CAD build for the part. Positions are in the model's coordinates, mm. A direction names the side the tool comes from. Give positions to 0.01 mm unless a question says otherwise; leave off trailing zeros. Write each loop counter-clockwise with the first axis right and the second up, starting at its lowest first coordinate (ties: lowest second). Pieces come first, ordered by that corner, then holes. Notation, with made-up numbers: (86.5, 88) - (99.5, 88) arc R9 cw to (99.5, 93) - close; hole circle Ø8 at (51, 25.5). An arc over 180 degrees is marked (long way). Write item = value, one per line. Start each with the question number.
```python
from build123d import *

# Parameters (mm, degrees)
SKETCH3_R                 = 2.75
BOSS_EXTRUDE1_DEPTH       = 6
BOSS_EXTRUDE1_2_DEPTH     = 6
BOSS_EXTRUDE1_3_DEPTH     = 6
BOSS_EXTRUDE1_4_DEPTH     = 6
SKETCH4_W                 = 43
SKETCH4_H                 = 86
BOSS_EXTRUDE2_DEPTH       = 2.5
SKETCH5_R                 = 2.75
BOSS_EXTRUDE3_DEPTH       = 10
LPATTERN1_COUNT           = 2
LPATTERN1_PITCH           = 37
LPATTERN2_COUNT           = 2
LPATTERN2_PITCH           = 37
LPATTERN2_COPY_1_SKETCH_R = 2.75
LPATTERN2_COPY_1_DEPTH    = 10
SKETCH6_W                 = 87
SKETCH6_H                 = 86
BOSS_EXTRUDE4_DEPTH       = 2.5
BOSS_EXTRUDE5_DEPTH       = 2
SKETCH12_W                = 4
SKETCH12_H                = 8
CUT_EXTRUDE1_DEPTH        = 4
SKETCH14_R                = 0.85
CUT_EXTRUDE2_DEPTH        = 4.5
LPATTERN3_COUNT           = 2
LPATTERN3_PITCH           = 46.5
BOSS_EXTRUDE6_DEPTH       = 35
SKETCH18_W                = 2
SKETCH18_H                = 35
BOSS_EXTRUDE7_DEPTH       = 18.5
SKETCH19_W                = 32.48
SKETCH19_H                = 17.04
BOSS_EXTRUDE8_DEPTH       = 10
SKETCH20_W                = 8.16
SKETCH20_H                = 13.04
CUT_EXTRUDE3_DEPTH        = 10
SKETCH21_W                = 1.1
SKETCH21_H                = 86
CUT_EXTRUDE4_DEPTH        = 10
FILLET2_R                 = 2
FILLET4_R                 = 20
BOSS_EXTRUDE9_DEPTH       = 2.5
SKETCH24_W                = 10
SKETCH24_H                = 20
BOSS_EXTRUDE10_DEPTH      = 30
SKETCH25_R                = 5
CUT_EXTRUDE6_DEPTH        = 30
FILLET6_R                 = 10
FILLET8_R                 = 2
SKETCH27_W                = 20
SKETCH27_H                = 20.130693805
CUT_EXTRUDE7_DEPTH        = 22.5
CUT_EXTRUDE10_DEPTH       = 7.5
CUT_EXTRUDE10_DEPTH_BACK  = 210.5
SKETCH28_W                = 79.126815109
SKETCH28_H                = 112.332596714
SKETCH29_R                = 1.25
CUT_EXTRUDE11_DEPTH       = 19.5
SKETCH30_W                = 10
SKETCH30_H                = 5
CUT_EXTRUDE12_DEPTH       = 4.5
FILLET9_R                 = 5
FILLET9_OF_MIRROR5_R      = 5
FILLET11_R                = 1


with BuildPart() as part:
    # Sketch3 → Boss-Extrude1 (new body)
    with BuildSketch(Plane.XY):
        with Locations((-25, -3)):
            Circle(SKETCH3_R)
    boss_extrude1 = extrude(amount=BOSS_EXTRUDE1_DEPTH)



with BuildPart() as body_2:
    # Sketch3 → Boss-Extrude1 2 (new body)
    with BuildSketch(Plane.XY):
        with Locations((-62, -3)):
            Circle(SKETCH3_R)
    boss_extrude1_2 = extrude(amount=BOSS_EXTRUDE1_2_DEPTH)


with BuildPart() as body_3:
    # Sketch3 → Boss-Extrude1 3 (new body)
    with BuildSketch(Plane.XY):
        with Locations(Location((-25, -40, 0), (0, 0, 180))):
            Circle(SKETCH3_R)
    boss_extrude1_3 = extrude(amount=BOSS_EXTRUDE1_3_DEPTH)


with BuildPart() as body_4:
    # Sketch3 → Boss-Extrude1 4 (new body)
    with BuildSketch(Plane.XY):
        with Locations(Location((-62, -40, 0), (0, 0, 180))):
            Circle(SKETCH3_R)
    boss_extrude1_4 = extrude(amount=BOSS_EXTRUDE1_4_DEPTH)


with BuildPart() as part_1:
    add(part.part)

    add(body_2.part)  # Boss-Extrude2 merges body 2

    add(body_3.part)  # Boss-Extrude2 merges body 3

    add(body_4.part)  # Boss-Extrude2 merges body 4
    # Sketch4 → Boss-Extrude2 (add)
    with BuildSketch(Plane.XY):
        with Locations((-43.5, 0)):
            Rectangle(SKETCH4_W, SKETCH4_H)
    extrude(amount=-BOSS_EXTRUDE2_DEPTH)

    # Mirror4: Boss-Extrude1, Boss-Extrude1 2, Boss-Extrude1 3, Boss-Extrude1 4 across plane
    add(boss_extrude1.mirror(Plane.ZX))
    add(boss_extrude1_2.mirror(Plane.ZX))
    add(boss_extrude1_3.mirror(Plane.ZX))
    add(boss_extrude1_4.mirror(Plane.ZX))

    # Sketch5 → Boss-Extrude3 (add)
    with BuildSketch(Plane.XY.offset(6)):
        with Locations((-25, 40)):
            Circle(SKETCH5_R)
    boss_extrude3 = extrude(amount=BOSS_EXTRUDE3_DEPTH)

    # LPattern1: Boss-Extrude3 ×2
    with Locations(*[(-i * LPATTERN1_PITCH, 0, 0) for i in range(1, LPATTERN1_COUNT)]):
        add(boss_extrude3)

    # LPattern2: Boss-Extrude3 ×2
    with Locations(*[(0, -i * LPATTERN2_PITCH, 0) for i in range(1, LPATTERN2_COUNT)]):
        add(boss_extrude3)

    # LPattern2 copy 1 sketch → LPattern2 copy 1 (add)
    with BuildSketch(Plane(origin=(-37, -37, 6), x_dir=(1, 0, 0), z_dir=(0, 0, 1))):
        with Locations((-25, 40)):
            Circle(LPATTERN2_COPY_1_SKETCH_R)
    extrude(amount=LPATTERN2_COPY_1_DEPTH)

    # Sketch6 → Boss-Extrude4 (add)
    with BuildSketch(Plane.XY):
        with Locations((21.5, 0)):
            Rectangle(SKETCH6_W, SKETCH6_H)
    extrude(amount=-BOSS_EXTRUDE4_DEPTH)

    # Sketch11 → Boss-Extrude5 (add, symmetric)
    with BuildSketch(Plane(origin=(-6, 0, 0), x_dir=(0, 0, -1), z_dir=(1, 0, 0))):
        Polygon((0, -43), (-40, -43), (-40, -39), (0, -18), align=None)
    boss_extrude5 = extrude(amount=BOSS_EXTRUDE5_DEPTH, both=True)

    # Sketch12 → Cut-Extrude1 (cut)
    with BuildSketch(Plane.ZY.offset(8)):
        with Locations((8, -32)):
            Rectangle(SKETCH12_W, SKETCH12_H)
    extrude(amount=-CUT_EXTRUDE1_DEPTH, mode=Mode.SUBTRACT)

    # Sketch14 → Cut-Extrude2 (cut)
    with BuildSketch(Plane.XZ.offset(43)):
        with Locations(Location((-6, 37, 0), (0, 0, 270))):
            Circle(SKETCH14_R)
        with Locations(Location((-6, 13.6, 0), (0, 0, 270))):
            Circle(SKETCH14_R)
    cut_extrude2 = extrude(amount=-CUT_EXTRUDE2_DEPTH, mode=Mode.SUBTRACT)

    # LPattern3: Boss-Extrude5, Cut-Extrude2 ×2
    with Locations(*[(i * LPATTERN3_PITCH, 0, 0) for i in range(1, LPATTERN3_COUNT)]):
        add(boss_extrude5)
        add(cut_extrude2, mode=Mode.SUBTRACT)

    # Sketch17 → Boss-Extrude6 (add)
    with BuildSketch(Plane.XY):
        Polygon((42.5, -41), (42.5, -43), (63.9, -43), (63.9, 25.4), (40.5, 25.4), (40.5, -18), (42.5, -18), (42.5, 23.4), (61.9, 23.4), (61.9, -41), align=None)
    extrude(amount=BOSS_EXTRUDE6_DEPTH)

    # Sketch18 → Boss-Extrude7 (add)
    with BuildSketch(Plane.XZ.offset(18)):
        with Locations((41.5, 17.5)):
            Rectangle(SKETCH18_W, SKETCH18_H)
    extrude(amount=BOSS_EXTRUDE7_DEPTH)

    # Sketch19 → Boss-Extrude8 (add)
    with BuildSketch(Plane.XY):
        with Locations((16.24, 8.52)):
            Rectangle(SKETCH19_W, SKETCH19_H)
    extrude(amount=BOSS_EXTRUDE8_DEPTH)

    # Sketch20 → Cut-Extrude3 (cut)
    with BuildSketch(Plane.XY.offset(10)):
        with Locations((6.08, 8.52)):
            Rectangle(SKETCH20_W, SKETCH20_H)
        with Locations((16.24, 8.52)):
            Rectangle(SKETCH20_W, SKETCH20_H)
        with Locations((26.4, 8.52)):
            Rectangle(SKETCH20_W, SKETCH20_H)
    extrude(amount=-CUT_EXTRUDE3_DEPTH, mode=Mode.SUBTRACT)

    # Sketch21 → Cut-Extrude4 (cut)
    with BuildSketch(Plane.XY):
        with Locations((64.45, 0)):
            Rectangle(SKETCH21_W, SKETCH21_H)
    extrude(amount=-CUT_EXTRUDE4_DEPTH, mode=Mode.SUBTRACT)

    # Fillet2
    fillet2_edges = [part_1.edges().sort_by_distance(p)[0] for p in [
        (63.9, -43, 16.25),
        (63.9, 25.4, 17.5),
        (-65, -43, -1.25),
        (-65, 43, -1.25),
    ]]
    fillet(fillet2_edges, radius=FILLET2_R)

    # Fillet4
    fillet4_edges = [part_1.edges().sort_by_distance(p)[0] for p in [
        (63.9, 43, -1.25),
    ]]
    fillet(fillet4_edges, radius=FILLET4_R)

    # Sketch23 → Boss-Extrude9 (add)
    with BuildSketch(Plane(origin=(0, 0, -2.5), x_dir=(-1, 0, 0), z_dir=(0, 0, -1))):
        with BuildLine():
            Line((95.480174176, -10), (105, -10))
            Line((105, -10), (110, -10))
            Line((110, -10), (110, 10))
            Line((110, 10), (105, 10))
            Line((105, 10), (95.480174176, 10))
            add(Edge.make_bspline(
                [(95.480174176, 10), (68.262963787, 8.86232235), (65, 41)],
                knots=[0, 0, 0, 1, 1, 1], degree=2))
            Line((65, 41), (65, -41))
            add(Edge.make_bspline(
                [(95.480174176, -10), (68.262963787, -8.86232235), (65, -41)],
                knots=[0, 0, 0, 1, 1, 1], degree=2))
        make_face()
    extrude(amount=-BOSS_EXTRUDE9_DEPTH)

    # Sketch24 → Boss-Extrude10 (add)
    with BuildSketch(Plane.XY):
        with Locations((-105, 0)):
            Rectangle(SKETCH24_W, SKETCH24_H)
    extrude(amount=BOSS_EXTRUDE10_DEPTH)

    # Sketch25 → Cut-Extrude6 (cut)
    with BuildSketch(Plane.ZY.offset(110)):
        with Locations((20, 0)):
            Circle(SKETCH25_R)
    extrude(amount=-CUT_EXTRUDE6_DEPTH, mode=Mode.SUBTRACT)

    # Fillet6
    fillet6_edges = [part_1.edges().sort_by_distance(p)[0] for p in [
        (-100, 0, 0),
    ]]
    fillet(fillet6_edges, radius=FILLET6_R)

    # Fillet8
    fillet8_edges = [part_1.edges().sort_by_distance(p)[0] for p in [
        (-110, 10, 15),
        (-110, -10, 15),
    ]]
    fillet(fillet8_edges, radius=FILLET8_R)

    # Sketch27 → Cut-Extrude7 (cut)
    with BuildSketch(Plane(origin=(0, 0, -2.5), x_dir=(-1, 0, 0), z_dir=(0, 0, -1))):
        with Locations((100, -0.065346902)):
            Rectangle(SKETCH27_W, SKETCH27_H)
    extrude(amount=-CUT_EXTRUDE7_DEPTH, mode=Mode.SUBTRACT)


with BuildPart() as cut_extrude7_piece_1:
    # of the separate pieces the step leaves, piece 1, a body of its own (cut_extrude7_pieces)
    add(part_1.part.solids().sort_by_distance((-90, -10.130693805, -2.5))[0])

    # Sketch28 → Cut-Extrude10 (cut, two sides: drawn at the far end of the back side and taken through both)
    with BuildSketch(Plane.ZY.offset(90).offset(-CUT_EXTRUDE10_DEPTH_BACK)):
        with Locations((27.34304702, -0.64713832)):
            Rectangle(SKETCH28_W, SKETCH28_H)
    extrude(amount=CUT_EXTRUDE10_DEPTH + CUT_EXTRUDE10_DEPTH_BACK, mode=Mode.SUBTRACT)


with BuildPart() as cut_extrude7_piece_2:
    # of the separate pieces the step leaves, piece 2, a body of its own (cut_extrude7_pieces)
    add(part_1.part.solids().sort_by_distance((-108, 10, 20))[0])

    # Sketch29 → Cut-Extrude11 (cut)
    with BuildSketch(Plane(origin=(0, 0, 20), x_dir=(-1, 0, 0), z_dir=(0, 0, -1))):
        with Locations((105, 7.5)):
            Circle(SKETCH29_R)
    cut_extrude11 = extrude(amount=-CUT_EXTRUDE11_DEPTH, mode=Mode.SUBTRACT)

    # Sketch30 → Cut-Extrude12 (cut)
    with BuildSketch(Plane.XY.offset(30)):
        with Locations((-105, 7.5)):
            Rectangle(SKETCH30_W, SKETCH30_H)
    cut_extrude12 = extrude(amount=-CUT_EXTRUDE12_DEPTH, mode=Mode.SUBTRACT)

    # Fillet9
    # the kernel refuses this fillet: 5 mm, written as the material it takes off along each edge
    with BuildSketch(Plane(origin=(-122.437342964, 5, 30), x_dir=(0, -1, 0), z_dir=(1, 0, 0))) as fillet9_piece_1:
        with BuildLine():
            CenterArc((4.974937186, 5), FILLET9_R, 185.739170477, 84.260829523)
            Line((0, 4.5), (-0.099498744, 4.49))
            ThreePointArc((-0.099498744, 4.49), (-0.1, 2.25), (-0.1, 0))
            Line((-0.1, 0), (0, -0.1))
            Line((0, -0.1), (4.974937186, -0.1))
            Line((4.974937186, -0.1), (4.974937186, 0))
        make_face()
    extrude(amount=34.874685928, mode=Mode.SUBTRACT)

    # Mirror5: Cut-Extrude11, Cut-Extrude12 across plane
    add(cut_extrude11.mirror(Plane.ZX), mode=Mode.SUBTRACT)
    add(cut_extrude12.mirror(Plane.ZX), mode=Mode.SUBTRACT)

    # Fillet9 of Mirror5
    # the kernel refuses this fillet: 5 mm, written as the material it takes off along each edge
    with BuildSketch(Plane(origin=(-122.437342964, -5, 30), x_dir=(0, 0, -1), z_dir=(1, 0, 0))) as fillet9_of_mirror5_piece_1:
        with BuildLine():
            CenterArc((5, 4.974937186), FILLET9_OF_MIRROR5_R, 180, 84.260829523)
            Line((0, 4.974937186), (-0.1, 4.974937186))
            Line((-0.1, 4.974937186), (-0.1, 0))
            Line((-0.1, 0), (0, -0.1))
            ThreePointArc((0, -0.1), (2.25, -0.1), (4.49, -0.099498744))
            Line((4.49, -0.099498744), (4.5, 0))
        make_face()
    extrude(amount=34.874685928, mode=Mode.SUBTRACT)

    # Fillet11
    fillet11_edges = [cut_extrude7_piece_2.edges().sort_by_distance(p)[0] for p in [
        (-104, 10, 25.5),
        (-109.414213562, 9.414213562, 25.5),
        (-110, 6.5, 25.5),
        (-100, 7.5, 25.5),
        (-100, 3.379164781, 28.708099244),
        (-110, 0, 30),
        (-110, 3.379164781, 28.708099244),
        (-109.414213562, -9.414213562, 25.5),
        (-110, -6.5, 25.5),
        (-100, -7.5, 25.5),
        (-104, -10, 25.5),
        (-100, 0, 30),
        (-100, -3.379164781, 28.708099244),
        (-110, -3.379164781, 28.708099244),
    ]]
    fillet(fillet11_edges, radius=FILLET11_R)


solid = cut_extrude7_piece_2.part
```
1. Tool access for faces 4 (the flat face through (-105, 6, 25.5)), 5 (the cylindrical face through (-100.285, -7.039, 25.199)), 6 (the cylindrical face through (-109.699, -6.47, 25.215)): list every direction of +Z, -Z, +X, -X, +Y, -Y with a clear straight run to the whole face (end or side of a thin tool).
2. Cut at A-A (x = -105). Give the cut face in (y, z), then the cut area to 3 significant figures.
3. Cut at D-D (y = -5.75). Give the cut face in (x, z).
4. Mould opens along Y. For faces 1 (the flat face through (-104, 6, 20)), 2 (the cylindrical face through (-105.06, 3.42, 28.67)), 3 (the cylindrical face through (-106.155, 7.021, 22.712)) say: +Y half, -Y half, draft (parallel to the pull), parting line (faces both ways), or undercut.
5. Pin check, flat tips, straight feed: pin 1 Ø1.5 at (x, z) = (-108.5, 28) entering from +Y; pin 2 Ø3 at (x, y) = (-105, 7.5) entering from +Z; pin 3 Ø1.5 at (y, z) = (-7, 27.5) entering from +X. Stop position of each tip, or through.
6. Cut at C-C (x = -103.25). Give the cut face in (y, z), then the cut area to 3 significant figures.
7. Cut at B-B (y = 7.5). Give the cut face in (x, z).
8. Wall check: line 1 along Y through (x, z) = (-105, 23.05); line 2 along Y through (x, z) = (-105, 24); line 3 along Z through (x, y) = (-104.25, -6). Give the ranges that are in metal, low to high.
Output:
q1.face_4 = +Z, +X, -X, +Y
q1.face_5 = +Z, +X, -Y
q1.face_6 = +Z, -X, -Y
q2.outline = (-10, 20) - (-8.75, 20) - (-8.75, 25.5) - (-9, 25.5) arc R1 ccw to (-10, 24.5) - close; (-6.25, 20) - (-5, 20) arc R5 cw to (5, 20) - (6.25, 20) - (6.25, 25.5) - (5, 25.5) arc R5 ccw to (0.03, 30) - (-0.03, 30) arc R5 ccw to (-5, 25.5) - (-6.25, 25.5) - close; (8.75, 20) - (10, 20) - (10, 24.5) arc R1 ccw to (9, 25.5) - (8.75, 25.5) - close
q2.area = 77.3 mm2
q3.outline = (-110, 20) - (-100, 20) - (-100, 24.5) arc R1 ccw to (-101, 25.5) - (-109, 25.5) arc R1 ccw to (-110, 24.5) - close
q4.face_1 = draft
q4.face_2 = +Y half
q4.face_3 = undercut
q5.pin_1 = 4.49
q5.pin_2 = 25.5
q5.pin_3 = through
q6.outline = (-10, 20) - (-5, 20) arc R5 cw to (5, 20) - (10, 20) - (10, 24.5) arc R1 ccw to (9, 25.5) - (5, 25.5) arc R5 ccw to (0.03, 30) - (-0.03, 30) arc R5 ccw to (-5, 25.5) - (-9, 25.5) arc R1 ccw to (-10, 24.5) - close
q6.area = 105 mm2
q7.outline = (-110, 20) - (-106.25, 20) - (-106.25, 25.5) - (-109, 25.5) arc R1 ccw to (-110, 24.5) - close; (-103.75, 20) - (-100, 20) - (-100, 24.5) arc R1 ccw to (-101, 25.5) - (-103.75, 25.5) - close
q8.line_1 = -10 to -8.75, -6.25 to -3.96, 3.96 to 6.25, 8.75 to 10
q8.line_2 = -10 to -8.75, -6.25 to -3, 3 to 6.25, 8.75 to 10
q8.line_3 = 20 to 25.5
